Input: part model. Units: mm. Frame: model coordinates. Coordinates: 2 decimals unless noted, no trailing zeros. Write each loop counter-clockwise with the first axis right and the second up, starting at its lowest first coordinate (ties: lowest second). Pieces come first, ordered by that corner, then holes. Notation, with made-up numbers: (60, 10.25) - (102, 10.25) arc R6 ccw to (102, 15.25) - close; hole circle Ø5 at (71.5, 58.5). An arc over 180 degrees is marked (long way). Use a Markdown table: item, result. Add a question column.
Q1. Section query A-A (z = 5.75). Return the cut outline in (x, y), then the cut area to 3 significant figures.
Q2. Material intervals for probe 1 along Y at (x, z) = (0.25, 7); probe 2 along X at (y, z) = (-1, 2.25); probe 3 along Z at (x, y) = (-1.25, -2.75), sorted ascending. Write a range as from..to.
Q3. Section query B-B (z = 2). Return the cut outline in (x, y).
Q4. Pin query (flat end, axial travel): P1, Ø1.5, axis at y = 2, z = 4.5, coming from the -X side; P2, Ø2, axis at x = -2.5, z = 7.5, coming from the -Y side; P3, Ø2, axis at x = -1.5, y = -1, coming from the -Z side. Return the tip coordinate at first contact, or that it passes through.
from build123d import *

# Parameters (mm, degrees)
F0_R     = 1.5
F1_DEPTH = 7.5
F4_SIZE2 = 1.5
F4_SIZE  = 3


with BuildPart() as f1:
    # F0 (on Top) → F1 (new body)
    with BuildSketch(Plane.XY):
        Circle(F0_R)
    extrude(amount=F1_DEPTH)

    # F2 (on Front) → F3 (revolve)
    with BuildSketch(Plane.XZ):
        with BuildLine():
            Line((0, 9.6), (0, 7.5))
            Line((0, 7.5), (3.375, 7.5))
            ThreePointArc((3.375, 7.5), (1.966819, 8.998906), (0, 9.6))
        make_face()
    revolve(axis=Axis((0, 0, 8.55), (0, 0, 1)))

    # F4
    f4_edges = [f1.edges().sort_by_distance(p)[0] for p in [
        (-1.5, 0, 0),
    ]]
    chamfer(f4_edges, length=F4_SIZE, length2=F4_SIZE2)


solid = f1.part
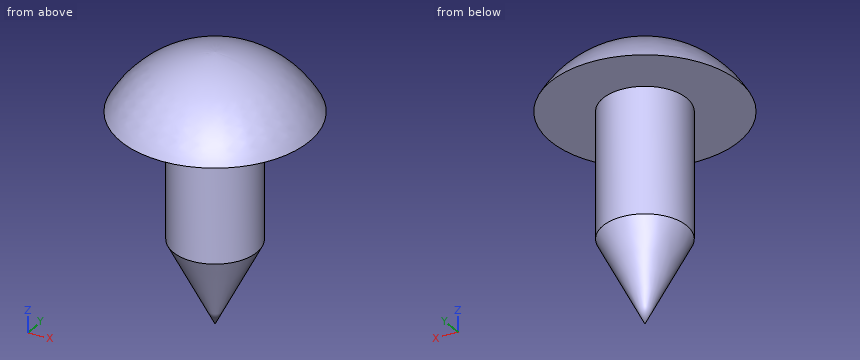
Values follow:
| question | item | result |
|---|---|---|
| 1 | outline | circle Ø3 at (0, 0) |
| 1 | area | 7.07 mm2 |
| 2 | probe 1 | -1.48..1.48 |
| 2 | probe 2 | -0.52..0.52 |
| 2 | probe 3 | 7.5..8.05 |
| 3 | outline | circle Ø2 at (0, 0) |
| 4 | P1 | x = -0.83 |
| 4 | P2 | y = -3.02 |
| 4 | P3 | z = 1.61 |
